Part model, mm, in its own coordinate system. A direction names the side the tool comes from. Give positions to 0.01 mm unless a question says otherwise; leave off trailing zeros. Order: outer loops, then holes, each group sorted by start corner. A loop starts at its lowest first (then second) coordinate and runs counter-clockwise, first axis right, second up.
1. Which spindle directions (+Z, -Z, +X, -X, +Y, -Y) get a long thin tool onto all of the face, cutting with end or side? Do faces 5 (the flat face through (-10, 10, 5)), 6 (the flat face through (10, 9.75, 3.85)), 7 (the flat face through (0.55, 10, 6)). Say none if no direction does.
2. Slice it at A-A on z = 3.9. List the corners of the cut face in (x, y) (3 decimals).
3. Slice it at C-C on z = 1. List the corners of the cut face in (x, y) (3 decimals).
4. Probe line 1 (X direction, y = 10.5, z = 6.75); line 2 (X direction, y = 0, z = 8.75) (3 decimals); line 3 (Y direction, x = 8, z = 3.9). List the from-to ranges inside material, lowest first.
5. Mould opens along Y. For faces 1 (the cylindrical face through (-17.16, -2.44, 3.48)), 2 (the cylindrical face through (-5.341, 9.936, 4.225)), 3 (the flat face through (6, 12, 7.8)), 4 (the flat face through (-14.39, 6.55, 3.85)) say: +Y half, -Y half, draft (parallel to the pull), parting line (faces both ways), or undercut.
6. Slice it at B-B on y = 0. List the corners of the cut face in (x, z) (3 decimals).
7. Drop flat-ended pins along their axis: pin 1 Ø2.5 at (y, z) = (10.5, 5.5) entering from -X; pin 2 Ø12 at (x, y) = (17, -6.5) entering from +Z; pin 3 Ø1.5 at (y, z) = (3.5, 10) entering from -X. Give the stop position or say it passes through.
8. Slice it at D-D on x = -17.7. List the corners of the cut face in (y, z), and give its area (3 significant figures).
from build123d import *

# Parameters (mm, degrees)
CROQUIS1_R              = 12.5
CROQUIS1_R_2            = 5.925
SALIENTE_EXTRUIR1_DEPTH = 12.8
CROQUIS2_R              = 5.925
SALIENTE_EXTRUIR2_DEPTH = 7.8
CROQUIS3_R              = 2.5
CORTAR_EXTRUIR1_DEPTH   = 7.8
CORTAR_EXTRUIR2_DEPTH   = 13
REDONDEO1_R             = 1
CORTAR_EXTRUIR3_START   = -20
CROQUIS5_R              = 1.5
CORTAR_EXTRUIR3_DEPTH   = 20
REDONDEO2_R             = 0.5
CHAFL_N1_SIZE           = 0.75


with BuildPart() as part:
    # Croquis1 → Saliente-Extruir1 (new body)
    with BuildSketch(Plane.XY):
        Circle(CROQUIS1_R)
        Circle(CROQUIS1_R_2, mode=Mode.SUBTRACT)
    extrude(amount=SALIENTE_EXTRUIR1_DEPTH)

    # Croquis2 → Saliente-Extruir2 (add)
    with BuildSketch(Plane(origin=(0, 0, 0), x_dir=(-1, 0, 0), z_dir=(0, 0, -1))):
        with BuildLine():
            Line((-6.439548023, -12.318369262), (-20.340677966, -5.051417611))
            ThreePointArc((-20.340677966, -5.051417611), (-23.348755649, 0.76260056), (-18.906641236, 5.570818336))
            Line((-18.906641236, 5.570818336), (-10, 7.5))
            Line((-10, 7.5), (-10, 13.9))
            Line((-10, 13.9), (10, 13.9))
            Line((10, 13.9), (10, 7.5))
            Line((10, 7.5), (18.906641236, 5.570818336))
            ThreePointArc((18.906641236, 5.570818336), (23.348755649, 0.76260056), (20.340677966, -5.051417611))
            Line((20.340677966, -5.051417611), (6.439548023, -12.318369262))
            ThreePointArc((6.439548023, -12.318369262), (0, -13.9), (-6.439548023, -12.318369262))
        make_face()
        Circle(CROQUIS2_R, mode=Mode.SUBTRACT)
    extrude(amount=-SALIENTE_EXTRUIR2_DEPTH)

    # Croquis3 → Cortar-Extruir1 (cut)
    with BuildSketch(Plane(origin=(0, 0, 0), x_dir=(-1, 0, 0), z_dir=(0, 0, -1))):
        with Locations((-17.7, 0)):
            Circle(CROQUIS3_R)
        with Locations((17.7, 0)):
            Circle(CROQUIS3_R)
    extrude(amount=-CORTAR_EXTRUIR1_DEPTH, mode=Mode.SUBTRACT)

    # Croquis4 → Cortar-Extruir2 (cut)
    with BuildSketch(Plane(origin=(0, 0, 0), x_dir=(-1, 0, 0), z_dir=(0, 0, -1))):
        with BuildLine():
            Line((0.55, 13.9), (-0.55, 13.9))
            Line((-0.55, 13.9), (-0.55, 5.899417344))
            ThreePointArc((-0.55, 5.899417344), (0, 5.925), (0.55, 5.899417344))
            Line((0.55, 5.899417344), (0.55, 13.9))
        make_face()
    extrude(amount=-CORTAR_EXTRUIR2_DEPTH, mode=Mode.SUBTRACT)

    # Redondeo1
    redondeo1_edges = [part.edges().sort_by_distance(p)[0] for p in [
        (0, -12.5, 12.8),
    ]]
    fillet(redondeo1_edges, radius=REDONDEO1_R)

    # Croquis5 → Cortar-Extruir3 (cut)
    with BuildSketch(Plane(origin=(10, 0, 0), x_dir=(0, 0, -1), z_dir=(1, 0, 0)).offset(CORTAR_EXTRUIR3_START)):
        with Locations((-3.9, 11.4)):
            Circle(CROQUIS5_R)
    extrude(amount=CORTAR_EXTRUIR3_DEPTH, mode=Mode.SUBTRACT)

    # Redondeo2
    redondeo2_edges = [part.edges().sort_by_distance(p)[0] for p in [
        (10, 13.9, 3.9),
        (-10, 13.9, 3.9),
    ]]
    fillet(redondeo2_edges, radius=REDONDEO2_R)

    # Chaflán1
    chafl_n1_edges = [part.edges().sort_by_distance(p)[0] for p in [
        (20.2, 0, 7.8),
        (-15.2, 0, 7.8),
    ]]
    chamfer(chafl_n1_edges, length=CHAFL_N1_SIZE)


solid = part.part
Data:
1. face 5: +Z, -Z, -X, +Y
1. face 6: +Z, -Z, +X, +Y
1. face 7: +Z, -Z, +Y
2. outline: (-20.341, -5.051) - (-6.44, -12.318) arc R13.9 ccw to (6.44, -12.318) - (20.341, -5.051) arc R5.7 ccw to (18.907, 5.571) - (10, 7.5) - (10, 9.9) - (0.55, 9.9) - (0.55, 5.899) arc R5.925 cw (long way) to (-0.55, 5.899) - (-0.55, 9.9) - (-10, 9.9) - (-10, 7.5) - (-18.907, 5.571) arc R5.7 ccw to start; (-10, 12.9) - (-0.55, 12.9) - (-0.55, 13.9) - (-9.5, 13.9) arc R0.5 ccw to (-10, 13.4) - close; (0.55, 12.9) - (10, 12.9) - (10, 13.4) arc R0.5 ccw to (9.5, 13.9) - (0.55, 13.9) - close; hole circle Ø5 at (-17.7, 0); hole circle Ø5 at (17.7, 0)
3. outline: (-20.341, -5.051) - (-6.44, -12.318) arc R13.9 ccw to (6.44, -12.318) - (20.341, -5.051) arc R5.7 ccw to (18.907, 5.571) - (10, 7.5) - (10, 13.4) arc R0.5 ccw to (9.5, 13.9) - (0.55, 13.9) - (0.55, 5.899) arc R5.925 cw (long way) to (-0.55, 5.899) - (-0.55, 13.9) - (-9.5, 13.9) arc R0.5 ccw to (-10, 13.4) - (-10, 7.5) - (-18.907, 5.571) arc R5.7 ccw to start; hole circle Ø5 at (-17.7, 0); hole circle Ø5 at (17.7, 0)
4. line 1: x = -10 to -0.55, 0.55 to 10
4. line 2: x = -12.5 to -5.925, 5.925 to 12.5
4. line 3: y = -11.5 to 9.9, 12.9 to 13.9
5. face 1: undercut
5. face 2: undercut
5. face 3: draft
5. face 4: +Y half
6. outline: (-23.4, 0) - (-20.2, 0) - (-20.2, 7.05) - (-20.95, 7.8) - (-23.4, 7.8) - close; (-15.2, 0) - (-5.925, 0) - (-5.925, 12.8) - (-11.5, 12.8) arc R1 ccw to (-12.5, 11.8) - (-12.5, 7.8) - (-14.45, 7.8) - (-15.2, 7.05) - close; (5.925, 0) - (15.2, 0) - (15.2, 7.05) - (14.45, 7.8) - (12.5, 7.8) - (12.5, 11.8) arc R1 ccw to (11.5, 12.8) - (5.925, 12.8) - close; (20.2, 0) - (23.4, 0) - (23.4, 7.8) - (20.95, 7.8) - (20.2, 7.05) - close
7. pin 1: stops at x = -10
7. pin 2: stops at z = 12.51
7. pin 3: stops at x = -12.19
8. outline: (-6.43, 0) - (-2.5, 0) - (-2.5, 7.05) - (-3.25, 7.8) - (-6.43, 7.8) - close; (2.5, 0) - (5.83, 0) - (5.83, 7.8) - (3.25, 7.8) - (2.5, 7.05) - close
8. area: 56.1 mm2
